from build123d import *


with BuildPart() as part:
    # Sketch1 → Revolve1 (revolve)
    with BuildSketch(Plane.XY, mode=Mode.PRIVATE) as revolve1_sk:
        with BuildLine():
            Line((-3.175, 6.35), (-4.7625, 6.35))
            Line((-4.7625, 6.35), (-4.7625, 2.794))
            Line((-4.7625, 2.794), (-9.525, 2.794))
            Line((-9.525, 2.794), (-9.525, 9.525))
            Line((-9.525, 9.525), (-8.951630735, 9.525))
            ThreePointArc((-8.951630735, 9.525), (-8.660025959, 9.466996204), (-8.412815367, 9.301815367))
            Line((-8.412815367, 9.301815367), (-6.888815367, 7.777815367))
            ThreePointArc((-6.888815367, 7.777815367), (-6.35, 7.554630735), (-5.811184633, 7.777815367))
            Line((-5.811184633, 7.777815367), (-4.287184633, 9.301815367))
            ThreePointArc((-4.287184633, 9.301815367), (-4.039974041, 9.466996204), (-3.748369265, 9.525))
            Line((-3.748369265, 9.525), (-3.175, 9.525))
            Line((-3.175, 9.525), (-3.175, 6.35))
        make_face()
    revolve(revolve1_sk.sketch.rotate(Axis((0, 0, 0), (-1, 0, 0)), 90), axis=Axis((0, 0, 0), (-1, 0, 0)))


solid = part.part
Source: CAD feature listing. Evaluate the final solid. Frame: model axes, mm. Give positions to 0.01 mm unless a question says otherwise; leave off trailing zeros. Write each loop counter-clockwise with the first axis right and the second up, starting at its lowest first coordinate (ties: lowest second). Pieces come first, ordered by that corner, then holes. Notation, with made-up numbers: M 37.5,31.5 L 76.5,31.5 A10 ccw 76.5,38.5 Z; hole C 7,39 d10. An arc over 180 degrees is marked long. Return JSON: item names as keys, results as strings. Group by question number.
1) Draft query along Y for faces 1 (the face through (-9.525, -2.3, 2)), 2 (the face through (-9.23, 9.3, 2.06)), 3 (the face through (-3.98, 3.86, 5.04)), 4 (the face through (-4.762, 1, -3)). Return one class per face: released by +Y, released by -Y, zero draft, split by the parting line, or undercut.
2) Cut plane D-D, the plane x = -7.5. Output: boundary loops of the cut face in (y, z).
3) Cut plane C-C, the plane x = -3.5. Output: boundary loops of the cut face in (y, z) (3 decimals).
4) First-contact query: pin 1 Ø3 at (x, z) = (-7, 2) entering from +Y; pin 2 Ø3 at (y, z) = (-2.5, 0) entering from +X; pin 3 Ø10 at (y, z) = (3.5, 4) entering from +X (3 decimals). Flat tips, straight axial feed; report the tip coordinate or a pass-through.
5) Ray query, L1, parallel to Y at x = -3.6, z = 0 (3 decimals); L2, parallel to X at y = -3.75, z = 3 (1 decimal); L3, parallel to Z at x = -5.5, y = 2.5. Return the intervals inside material, ascending.
Data:
{
 "1": {"face 1": "zero draft", "face 2": "split by the parting line", "face 3": "undercut", "face 4": "undercut"},
 "2": {"outline": "C 0,0 d16.78; hole C 0,0 d5.59"},
 "3": {"outline": "C 0,0 d19.05; hole C 0,0 d12.7"},
 "4": {"pin 1": "stops at y = 9.2", "pin 2": "stops at x = -4.76", "pin 3": "stops at x = -3.175"},
 "5": {"L1": "y = -9.525 to -6.35, 6.35 to 9.525", "L2": "x = -9.5 to -4.8", "L3": "z = -7.69 to -1.25, 1.25 to 7.69"}
}
